```python
from build123d import *

# Parameters (mm, degrees)
F0_W     = 40
F0_H     = 40
F1_DEPTH = 50
F2_R     = 6
F3_DEPTH = 40
F5_DEPTH = 13
F6_DEPTH = 20


with BuildPart() as f1:
    # F0 (on Top) → F1 (new body)
    with BuildSketch(Plane.XY):
        Rectangle(F0_W, F0_H)
    extrude(amount=F1_DEPTH)

    # F2 (on face) → F3 (cut)
    with BuildSketch(Plane(origin=(0, 0, 0), x_dir=(1, 0, 0), z_dir=(0, 0, -1))):
        Circle(F2_R)
    extrude(amount=-F3_DEPTH, mode=Mode.SUBTRACT)

    # F4 (on face) → F5 (cut)
    with BuildSketch(Plane.XZ.offset(20)):
        with BuildLine():
            ThreePointArc((2.5, 35), (1.767766953, 36.767766953), (0, 37.5))
            ThreePointArc((0, 37.5), (-1.767766953, 33.232233047), (2.5, 35))
        make_face()
        with BuildLine():
            ThreePointArc((2.5, 15), (-1.767766953, 16.767766953), (0, 12.5))
            ThreePointArc((0, 12.5), (1.767766953, 13.232233047), (2.5, 15))
        make_face()
    extrude(amount=-F5_DEPTH, mode=Mode.SUBTRACT)

    # F6 (cut): a face of the model
    f6_faces = [f1.faces().sort_by_distance(p)[0] for p in [
        (0, 20, 25),
    ]]
    extrude(f6_faces, amount=-F6_DEPTH, mode=Mode.SUBTRACT)

    # F7: F1 across plane


with BuildPart() as f1_1:
    add(f1.part)
    add(f1.part.mirror(Plane.XZ))


solid = f1_1.part
```
Read the model definition and answer for the solid it produces. Units are mm, in the model's axes. A direction names the side the tool comes from. Coordinates: 2 decimals unless noted, no trailing zeros. Loops run counter-clockwise (first coordinate to the right, second up) from the corner with the lowest first, then second, coordinate; pieces in that order, holes last. Notation, with made-up numbers: (82.25, 89) -> (111.25, 89) arc R14 ccw to (111.25, 101) -> close; hole circle Ø1 at (12, 50.5). An arc over 180 degrees is marked (long way). Return JSON: item names as keys, results as strings.
Item 1: Find section C-C (y = 0). Determine the outline of the cut face in (x, z).
Answers:
{"outline": "(-20, 0) -> (-6, 0) -> (-6, 40) -> (6, 40) -> (6, 0) -> (20, 0) -> (20, 50) -> (-20, 50) -> close"}
Item 2: Find section B-B (z = 27). Determine the outline of the cut face in (x, y), plus the area to 3 significant figures.
Answers:
{"outline": "(-20, -20) -> (20, -20) -> (20, 20) -> (-20, 20) -> close; hole circle Ø12 at (0, 0)", "area": "1,490 mm2"}
Item 3: Find section A-A (y = -16). Determine the outline of the cut face in (x, z).
Answers:
{"outline": "(-20, 0) -> (20, 0) -> (20, 50) -> (-20, 50) -> close; hole circle Ø5 at (0, 15); hole circle Ø5 at (0, 35)"}
Item 4: Find the intervals of material crossed by probe 1 along Z at (x, y) = (0, 13); probe 2 along X at (y, z) = (13.75, 35); probe 3 along Y at (x, z) = (-0.5, 7), in increasing order.
Answers:
{"probe 1": "z = 0 to 12.5, 17.5 to 32.5, 37.5 to 50", "probe 2": "x = -20 to -2.5, 2.5 to 20", "probe 3": "y = -20 to -5.98, 5.98 to 20"}
Item 5: For a pull along Z with two mould halves and no side action, classify faces 1 (the flat face through (0, -7, 15)), 2 (the flat face through (-5, -5, 0)), 3 (the flat face through (-20, 0, 25)) as +Z half, -Z half, draft (parallel to the pull), parting line (faces both ways), or undercut.
Answers:
{"face 1": "undercut", "face 2": "-Z half", "face 3": "draft"}
Item 6: For faces 4 (the flat face through (0, -7, 35)), 5 (the flat face through (0, 7, 15)), 6 (the flat face through (0, 0, 50)), 7 (the flat face through (0, 20, 25)), 8 (the cylindrical face through (-6, 0, 20)), determine the directions among +Z, -Z, +X, -X, +Y, -Y from which every point of the face is accessible in a straight line to the end or side of a thin tool.
Answers:
{"face 4": "-Y", "face 5": "+Y", "face 6": "+Z, +X, -X, +Y, -Y", "face 7": "+Z, -Z, +X, -X, +Y", "face 8": "-Z"}
Item 7: Flat-ended cylindrical pins translate along their axes: P1, Ø11, axis at x = 0, y = 0, coming from the -Z side; P2, Ø1.5, axis at x = -1, z = 15.5, coming from the +Y side; P3, Ø3, axis at x = 0, z = 15, coming from the -Y side. Find the tip coordinate at first contact, or state that the pin passes through.
Answers:
{"P1": "stops at z = 40", "P2": "stops at y = 7", "P3": "stops at y = -7"}
